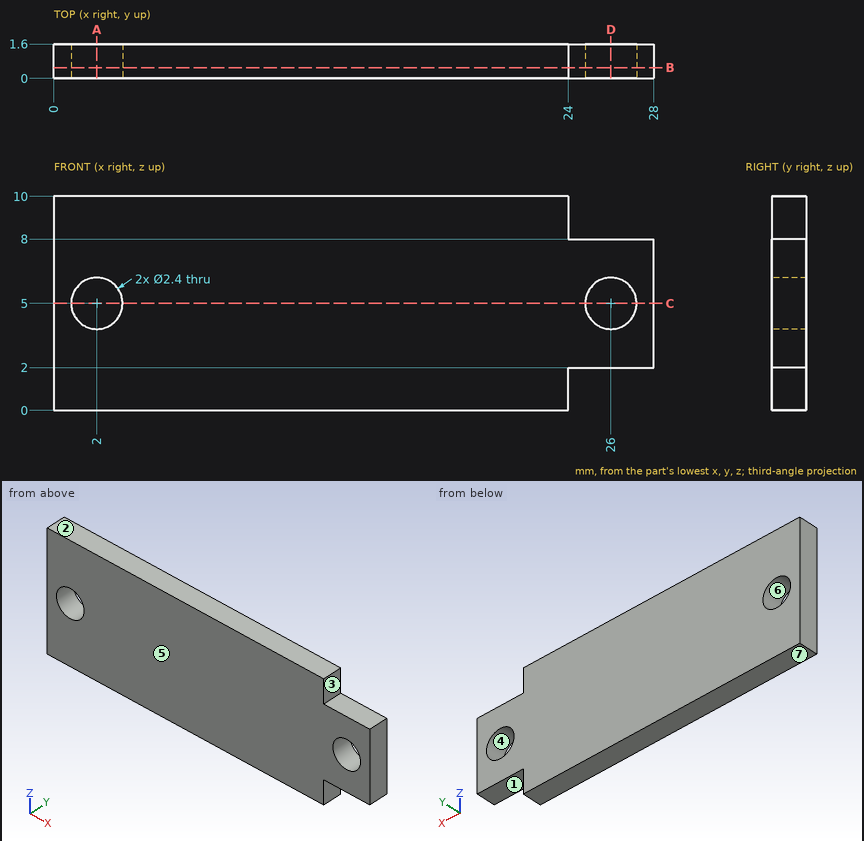
Design review of the part shown in the three views and the two pictorial views. Dimensions are in mm from the part's minimum x, y and z. A direction names the side the tool comes from. Round coordinates to 2 decimals unless told otherwise and drop trailing zeros. Loops run counter-clockwise (first coordinate to the right, second up) from the corner with the lowest first, then second, coordinate; pieces in that order, holes last. Notation, with made-up numbers: (-22, 79) - (2, 79) arc R23 ccw to (2, 118) - close; hole circle Ø10 at (-15.75, 81.5). An arc over 180 degrees is marked (long way). One line per item, written item: value. Start each with the question number.
Item 1: For L1, parallel to Z at x = 26, y = 0.8; L2, parallel to X at y = 0.65, z = 5; L3, parallel to Z at x = 2, y = 0.65, list the stretches that pass through material, from the lowest coordinate up.
Item 2: Take a section at B-B (y = 0.5). Give the boundary of the cut face in (x, z), plus the area to 3 significant figures.
Item 3: Clearance check with a flat-ended pin moving along its axis: pin 1 Ø1.4 at (x, z) = (2, 5) entering from -Y. State where the tip first meets the part, or that it passes through.
Item 4: The part is to be moulded in two halves that separate along Z. For the marked faces 4, 5, 6 and 7, say which applies: +Z half, -Z half, draft (parallel to the pull), parting line (faces both ways), or undercut.
Item 5: Take a section at C-C (z = 5). Give the boundary of the cut face in (x, y), plus the area to 3 significant figures.
Item 6: For the marked faces 1, 2 and 3, list the 3-axis set-ups (+Z, -Z, +X, -X, +Y, -Y) from which the entire face can be reached by the end or side of a thin tool; tool diameter is ignored.
Item 7: Take a section at A-A (x = 2). Give the boundary of the cut face in (y, z).
Item 8: Take a section at D-D (x = 26). Give the boundary of the cut face in (y, z).
Answer below:
1. L1: z = 2 to 3.8, 6.2 to 8
1. L2: x = 0 to 0.8, 3.2 to 24.8, 27.2 to 28
1. L3: z = 0 to 3.8, 6.2 to 10
2. outline: (0, 0) - (24, 0) - (24, 2) - (28, 2) - (28, 8) - (24, 8) - (24, 10) - (0, 10) - close; hole circle Ø2.4 at (2, 5); hole circle Ø2.4 at (26, 5)
2. area: 255 mm2
3. pin 1: passes through
4. face 4: undercut
4. face 5: draft
4. face 6: undercut
4. face 7: -Z half
5. outline: (0, 0) - (0.8, 0) - (0.8, 1.6) - (0, 1.6) - close; (3.2, 0) - (24.8, 0) - (24.8, 1.6) - (3.2, 1.6) - close; (27.2, 0) - (28, 0) - (28, 1.6) - (27.2, 1.6) - close
5. area: 37.1 mm2
6. face 1: -Z, +X, +Y, -Y
6. face 2: +Z, +X, -X, +Y, -Y
6. face 3: +Z, +X, +Y, -Y
7. outline: (0, 0) - (1.6, 0) - (1.6, 3.8) - (0, 3.8) - close; (0, 6.2) - (1.6, 6.2) - (1.6, 10) - (0, 10) - close
8. outline: (0, 2) - (1.6, 2) - (1.6, 3.8) - (0, 3.8) - close; (0, 6.2) - (1.6, 6.2) - (1.6, 8) - (0, 8) - close
